Could you check a few things on this model? Use its own coordinates, in mm. Face numbers are marked on the shaded views. A direction names the side the tool comes from. Coordinates: 2 decimals unless noted, no trailing zeros. Loops run counter-clockwise (first coordinate to the right, second up) from the corner with the lowest first, then second, coordinate; pieces in that order, holes last. Notation, with made-up numbers: M 44.25,11 L 78.25,11 A29 ccw 78.25,31 Z; hole C -19.5,29.25 d6. An arc over 180 degrees is marked long. Use one line per item in the form item = value. Start each with the question number.
```python
from build123d import *

# Parameters (mm, degrees)
SKETCH2_R           = 9.5
BOSS_EXTRUDE1_DEPTH = 6
CUT_EXTRUDE1_DEPTH  = 3.65
SKETCH4_R           = 2.5
CUT_EXTRUDE2_DEPTH  = 14.92201494
CUT_EXTRUDE4_DEPTH  = 3
SKETCH5_R           = 1.5
CUT_EXTRUDE5_DEPTH  = 15.71393897


with BuildPart() as part:
    # Sketch2 → Boss-Extrude1 (new body)
    with BuildSketch(Plane(origin=(0, 0, 0), x_dir=(1, 0, 0), z_dir=(0, 1, 0))):
        with Locations(Location((0, 0, 0), (0, 0, 270))):
            Circle(SKETCH2_R)
    extrude(amount=BOSS_EXTRUDE1_DEPTH)

    # Sketch3 → Cut-Extrude1 (cut)
    with BuildSketch(Plane(origin=(0, 6, 0), x_dir=(1, 0, 0), z_dir=(0, 1, 0))):
        Polygon((2.1975, -3.80618165), (4.395, 0), (2.1975, 3.80618165), (-2.1975, 3.80618165), (-4.395, 0), (-2.1975, -3.80618165), align=None)
    extrude(amount=-CUT_EXTRUDE1_DEPTH, mode=Mode.SUBTRACT)

    # Sketch4 → Cut-Extrude2 (cut, through all)
    with BuildSketch(Plane(origin=(0, 2.35, 0), x_dir=(1, 0, 0), z_dir=(0, 1, 0))):
        with Locations(Location((0, 0, 0), (0, 0, 270))):
            Circle(SKETCH4_R)
    extrude(amount=-CUT_EXTRUDE2_DEPTH, mode=Mode.SUBTRACT)

    # Sketch6 → Cut-Extrude4 (cut)
    with BuildSketch(Plane.XZ):
        Polygon((-2.598076211, -8.204916605), (0, -9.704916605), (2.598076211, -8.204916605), (2.598076211, -5.204916605), (0, -3.704916605), (-2.598076211, -5.204916605), align=None)
        Polygon((8.204916605, -2.598076211), (9.704916605, 0), (8.204916605, 2.598076211), (5.204916605, 2.598076211), (3.704916605, 0), (5.204916605, -2.598076211), align=None)
        Polygon((-8.204916605, 2.598076211), (-9.704916605, 0), (-8.204916605, -2.598076211), (-5.204916605, -2.598076211), (-3.704916605, 0), (-5.204916605, 2.598076211), align=None)
        Polygon((2.598076211, 8.204916605), (0, 9.704916605), (-2.598076211, 8.204916605), (-2.598076211, 5.204916605), (0, 3.704916605), (2.598076211, 5.204916605), align=None)
    extrude(amount=-CUT_EXTRUDE4_DEPTH, mode=Mode.SUBTRACT)

    # Sketch5 → Cut-Extrude5 (cut, through all)
    with BuildSketch(Plane(origin=(0, 6, 0), x_dir=(1, 0, 0), z_dir=(0, 1, 0))):
        with Locations(Location((6.5, 0, 0), (0, 0, 270))):
            Circle(SKETCH5_R)
        with Locations(Location((0, -6.5, 0), (0, 0, 270))):
            Circle(SKETCH5_R)
        with Locations(Location((-6.5, 0, 0), (0, 0, 270))):
            Circle(SKETCH5_R)
        with Locations(Location((0, 6.5, 0), (0, 0, 270))):
            Circle(SKETCH5_R)
    extrude(amount=-CUT_EXTRUDE5_DEPTH, mode=Mode.SUBTRACT)


solid = part.part
```
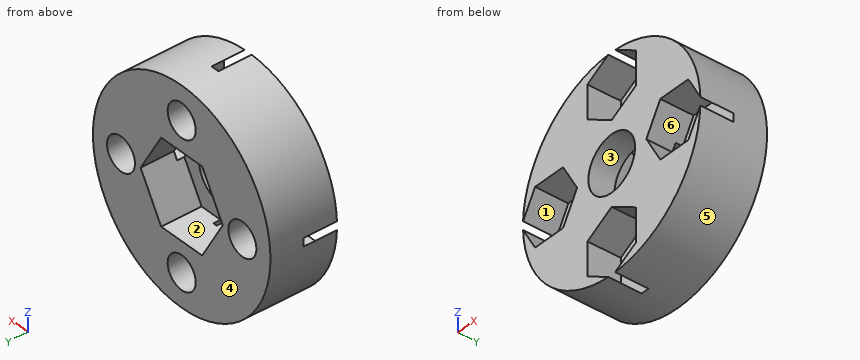
Item 1: Thinking about a two-plate mould opening in Z: for the marked faces 4, 5 and 6, which applies, pulls with the +Z half, pulls with the -Z half, needs draft (parallel to the pull), parting line crosses it, or undercut?
Item 2: I want a section at D-D (x = 7). Write out the boundary of the cut face in (y, z), plus the area to 3 significant figures.
Item 3: For the marked faces 1, 2 and 3, which set-ups out of +Z, -Z, +X, -X, +Y, -Y let a thin tool reach every point of the face, with its end or its side?
Item 4: I'm going to push flat-ended pins straight in: P1, Ø3.5, axis at x = 6, y = 1.5, coming from the -Z side; P2, Ø5.5, axis at x = 7, z = 1, coming from the -Y side; P3, Ø1, axis at y = 0.5, z = -1, coming from the -X side; P4, Ø2, axis at x = 1.5, y = 2, coming from the -Z side. Where does each tip first touch, or does it pass through?
Item 5: I want a section at A-A (y = 5.15). Write out the boundary of the cut face in (x, z) (1 decimal).
Item 6: Please list where these lines run through material, in increasing order: line 1 along Z through (x, y) = (-1, 2); line 2 along X through (y, z) = (3.65, -6.5); line 3 along X through (y, z) = (0.8, -8.5).
Item 7: I want a section at B-B (z = 7.75). Write out the boundary of the cut face in (x, y).
Worked answers:
q1.face_4 = needs draft
q1.face_5 = parting line crosses it
q1.face_6 = undercut
q2.outline = M 0,-6.42 L 6,-6.42 L 6,-1.41 L 3,-1.41 L 3,-2.6 L 0,-2.6 Z; M 0,2.6 L 3,2.6 L 3,1.41 L 6,1.41 L 6,6.42 L 0,6.42 Z
q2.area = 53.0 mm²
q3.face_1 = -Y
q3.face_2 = +Y
q3.face_3 = +Y, -Y
q4.P1 = -8.5
q4.P2 = 0
q4.P3 = -9.49
q4.P4 = -9.49
q5.outline = C 0,0 d19; hole C -6.5,0 d3; hole M -4.4,0 L -2.2,-3.8 L 2.2,-3.8 L 4.4,0 L 2.2,3.8 L -2.2,3.8 Z; hole C 0,-6.5 d3; hole C 0,6.5 d3; hole C 6.5,0 d3
q6.line_1 = -9.45 to -9.13, -4.28 to -2.29, 2.29 to 4.28, 9.13 to 9.45
q6.line_2 = -6.93 to -1.5, 1.5 to 6.93
q6.line_3 = -4.24 to -2.09, 2.09 to 4.24
q7.outline = M -5.49,0 L -2.6,0 L -2.6,3 L -0.83,3 L -0.83,6 L -5.49,6 Z; M 0.83,3 L 2.6,3 L 2.6,0 L 5.49,0 L 5.49,6 L 0.83,6 Z
